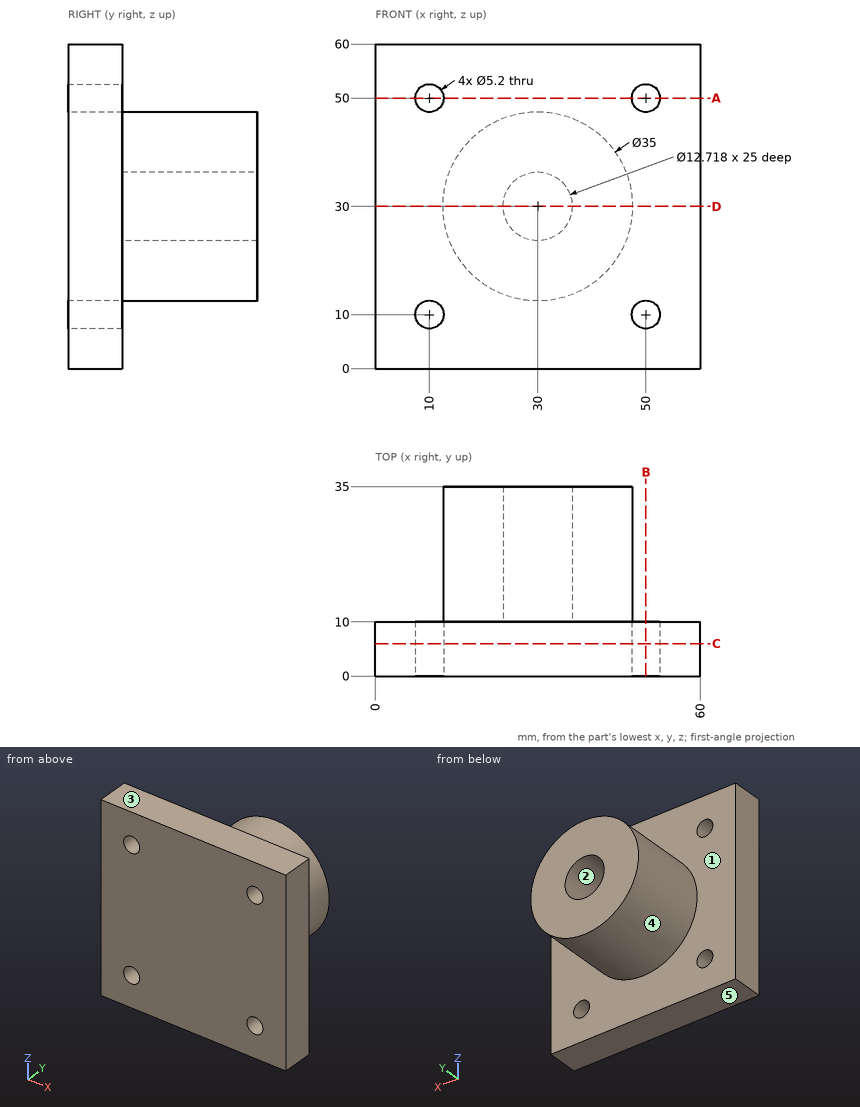
For this review, use the dimensioned drawing (mm, ordinates from the lowest corner) and the shaded views. A direction names the side the tool comes from. Give positions to 0.01 mm unless a question says otherwise; leave off trailing zeros. Loops run counter-clockwise (first coordinate to the right, second up) from the corner with the lowest first, then second, coordinate; pieces in that order, holes last. Notation, with made-up numbers: (-28.5, -39.75) -> (-5.5, -39.75) arc R30 ccw to (-5.5, -10.75) -> close; hole circle Ø7 at (65, 2.5). An arc over 180 degrees is marked (long way). One line per question, with ' | ' between items. Start each with the question number.
(1) We need section A-A (z = 50). State the section outline as (x, y) points.
(2) Draft analysis for pull direction Z (two halves, no side actions). For the marked faces 1, 2 and 3, state which applies: +Z half, -Z half, draft (parallel to the pull), parting line (faces both ways), or undercut.
(3) Insertion check: P1, Ø2, axis at x = 44, y = 25.5, coming from the +Z side (1 decimal); P2, Ø1, axis at x = 14, y = 23, coming from the +Z side (1 decimal); P3, Ø6, axis at x = 50, z = 10, coming from the +Y side. Each pin has a flat end and moves straight along its axis. Give the tip position at first contact, or say it passes through.
(4) We need section D-D (z = 30). State the section outline as (x, y) points, and give its area (3 significant figures).
(5) For line 1 (X direction, y = 4.5, z = 50); line 2 (Y direction, x = 7, z = 8); line 3 (X direction, y = 15, z = 39), list the stretches that pass through material, from the lowest coordinate up.
(6) For the marked faces 4 and 5, list the 3-axis set-ups (+Z, -Z, +X, -X, +Y, -Y) from which the entire face can be reached by the end or side of a thin tool; tool diameter is ignored.
(7) We need section B-B (x = 50). State the section outline as (y, z) points.
(8) We need section C-C (y = 6). State the section outline as (x, z) points, and give its area (4 significant figures).
The answers:
1) outline: (0, 0) -> (7.4, 0) -> (7.4, 10) -> (0, 10) -> close; (12.6, 0) -> (47.4, 0) -> (47.4, 10) -> (12.6, 10) -> close; (52.6, 0) -> (60, 0) -> (60, 10) -> (52.6, 10) -> close
2) face 1: draft | face 2: undercut | face 3: +Z half
3) P1: stops at z = 41.7 | P2: stops at z = 38.1 | P3: stops at y = 10
4) outline: (0, 0) -> (60, 0) -> (60, 10) -> (47.5, 10) -> (47.5, 35) -> (36.36, 35) -> (36.36, 10) -> (23.64, 10) -> (23.64, 35) -> (12.5, 35) -> (12.5, 10) -> (0, 10) -> close | area: 1,160 mm^2
5) line 1: x = 0 to 7.4, 12.6 to 47.4, 52.6 to 60 | line 2: y = 0 to 10 | line 3: x = 14.99 to 45.01
6) face 4: +Y | face 5: -Z, +X, -X, +Y, -Y
7) outline: (0, 0) -> (10, 0) -> (10, 7.4) -> (0, 7.4) -> close; (0, 12.6) -> (10, 12.6) -> (10, 47.4) -> (0, 47.4) -> close; (0, 52.6) -> (10, 52.6) -> (10, 60) -> (0, 60) -> close
8) outline: (0, 0) -> (60, 0) -> (60, 60) -> (0, 60) -> close; hole circle Ø5.2 at (10, 10); hole circle Ø5.2 at (10, 50); hole circle Ø5.2 at (50, 10); hole circle Ø5.2 at (50, 50) | area: 3,515 mm^2
